from build123d import *

# Parameters (mm, degrees)
BOSS_EXTRUDE1_DEPTH = 5
SKETCH2_W           = 5
SKETCH2_H           = 90
SKETCH2_H_2         = 40
SKETCH2_W_2         = 35
SKETCH2_H_3         = 5
CUT_EXTRUDE1_DEPTH  = 10
CUT_EXTRUDE2_DEPTH  = 10
FILLET1_R           = 1
FILLET2_R           = 10
CUT_EXTRUDE3_DEPTH  = 10


with BuildPart() as part:
    # Sketch1 → Boss-Extrude1 (new body)
    with BuildSketch(Plane.XY):
        Polygon((80, 33.22), (20, 33.22), (20, 600), (80, 600), (80, 570.05), (84.9, 570.05), (84.9, 449.95), (80, 449.95), (80, 390.05), (84.9, 390.05), (84.9, 269.95), (80, 269.95), (80, 210.05), (84.9, 210.05), (84.9, 89.95), (80, 89.95), align=None)
    extrude(amount=BOSS_EXTRUDE1_DEPTH)

    # Sketch2 → Cut-Extrude1 (cut)
    with BuildSketch(Plane.XY.offset(5)):
        Polygon((67, 370.417424305), (62.417424305, 368.417424305), (70.417424305, 350.087121525), (75, 352.087121525), align=None)
        Polygon((73.902811841, 226.418897298), (51.258042728, 139.314279557), (56.097188159, 138.056236829), (78.741957272, 225.16085457), align=None)
        with Locations((52.33914543, 83.217091399)):
            Rectangle(SKETCH2_W, SKETCH2_H)
        with Locations((42.33914543, 119.314279557)):
            Rectangle(SKETCH2_W, SKETCH2_H_2)
        with Locations((42.5, 377.5)):
            Rectangle(SKETCH2_W_2, SKETCH2_H_3)
    extrude(amount=-CUT_EXTRUDE1_DEPTH, mode=Mode.SUBTRACT)

    # Sketch3 → Cut-Extrude2 (cut)
    with BuildSketch(Plane.XY.offset(5)):
        Polygon((20, 395), (65, 600), (1.513631165, 616.08755832), align=None)
        Polygon((45, 33.22), (20, 58.22), (13.452472792, 20.556075169), align=None)
    extrude(amount=-CUT_EXTRUDE2_DEPTH, mode=Mode.SUBTRACT)

    # Fillet1
    fillet1_edges = [part.edges().sort_by_distance(p)[0] for p in [
        (84.9, 570.05, 2.5),
        (84.9, 449.95, 2.5),
        (84.9, 390.05, 2.5),
        (84.9, 269.95, 2.5),
        (84.9, 210.05, 2.5),
        (84.9, 89.95, 2.5),
    ]]
    fillet(fillet1_edges, radius=FILLET1_R)

    # Fillet2
    fillet2_edges = [part.edges().sort_by_distance(p)[0] for p in [
        (20, 395, 2.5),
        (65, 600, 2.5),
        (45, 33.22, 2.5),
        (20, 58.22, 2.5),
    ]]
    fillet(fillet2_edges, radius=FILLET2_R)

    # Sketch4 → Cut-Extrude3 (cut)
    with BuildSketch(Plane.XY.offset(5)):
        Polygon((60.059418786, 577.492907801), (64.943140501, 576.420871327), (60.654994605, 556.885984463), (55.771272889, 557.958020937), align=None)
    extrude(amount=-CUT_EXTRUDE3_DEPTH, mode=Mode.SUBTRACT)


solid = part.part
Design review of the part built by this model. Coordinates are the model's own, in mm. A direction names the side the tool comes from. Round coordinates to 2 decimals unless told otherwise and drop trailing zeros. Write each loop counter-clockwise with the first axis right and the second up, starting at its lowest first coordinate (ties: lowest second). Pieces come first, ordered by that corner, then holes. Notation, with made-up numbers: (2.5, 21) - (58.5, 21) arc R22 ccw to (58.5, 36) - close; hole circle Ø6 at (-37.75, 64). An arc over 180 degrees is marked (long way). Return JSON: item names as keys, results as strings. Group by question number.
Item 1: We need section A-A on y = 73.5. Write out the cut boundary in (x, z).
Item 2: For probe 1 along Y at (x, z) = (80.5, 1.85); probe 2 along X at (y, z) = (65.5, 3.7); probe 3 along X at (y, z) = (189.5, 4.55), list the stretches that pass through material, from the lowest coordinate up. Write a range as [from, to].
Item 3: Machinability: for faces 5 (the face through (53, 321, 0)), 6 (the face through (67.26, 181, 2.54)), which of the approach directions +Z, -Z, +X, -X, +Y, -Y give a long, thin tool a straight path to every point of the face, cutting with its end or side? Answer none if there is none.
Item 4: We need section B-B on x = 35. Write out the cut boundary in (y, z), and give its area (3 significant figures).
Item 5: The part is to be moulded in two halves that separate along Y. For faces 1 (the face through (37.753, 475.875, 2.535)), 2 (the face through (53, 321, 5)), 3 (the face through (62.74, 183.48, 2.54)), 4 (the face through (32.63, 45.59, 2.54)), say which applies: pulls with the +Y half, pulls with the -Y half, needs draft (parallel to the pull), parting line crosses it, or undercut.
Item 6: Insertion check: P1, Ø2.5, axis at y = 408, z = 2, coming from the +X side; P2, Ø3, axis at x = 36.5, z = 4.5, coming from the -Y side; P3, Ø1.2, axis at x = 82.5, z = 2.5, coming from the -Y side. Each pin has a flat end and moves straight along its axis. Give the tip position at first contact, or say it passes through.
Item 7: We need section D-D on y = 535.5. Write out the cut boundary in (x, z).
Item 8: We need section C-C on z = 3.1. Give the number of separate pieces and of enclosed holes in the cut face, and give its area (3 significant figures).
Model answer:
{
 "1": {"outline": "(20, 0) - (49.84, 0) - (49.84, 5) - (20, 5) - close; (54.84, 0) - (80, 0) - (80, 5) - (54.84, 5) - close"},
 "2": {"probe 1": "y = [89.95, 210.05], [269.95, 390.05], [449.95, 570.05]", "probe 2": "x = [20, 49.84], [54.84, 80]", "probe 3": "x = [20, 64.3], [69.47, 84.9]"},
 "3": {"face 5": "-Z, +X, -X, +Y, -Y", "face 6": "+Z, -Z"},
 "4": {"outline": "(43.22, 0) - (375, 0) - (375, 5) - (43.22, 5) - close; (380, 0) - (463.33, 0) - (463.33, 5) - (380, 5) - close", "area": "2,080 mm²"},
 "5": {"face 1": "pulls with the +Y half", "face 2": "needs draft", "face 3": "undercut", "face 4": "pulls with the -Y half"},
 "6": {"P1": "stops at x = 80", "P2": "stops at y = 40.22", "P3": "stops at y = 89.95"},
 "7": {"outline": "(50.84, 0) - (84.9, 0) - (84.9, 5) - (50.84, 5) - close"},
 "8": {"separate pieces": "1", "enclosed holes": "5", "area": "29,400 mm²"}
}
